```python
from build123d import *

# Parameters (mm, degrees)
AUFSATZ_LINEAR_AUSTRAGEN1_DEPTH = 5
VERRUNDUNG2_R                   = 2
SKIZZE7_R                       = 15
AUFSATZ_LINEAR_AUSTRAGEN3_DEPTH = 10
AUFSATZ_LINEAR_AUSTRAGEN5_DEPTH = 10
SCHNITT_LINEAR_AUSTRAGEN2_REACH = 17
SKIZZE9_R                       = 4
SCHNITT_LINEAR_AUSTRAGEN3_REACH = 7
SKIZZE10_R                      = 4


with BuildPart() as part:
    # Skizze1 → Aufsatz-Linear austragen1 (new body)
    with BuildSketch(Plane(origin=(0, 0, 0), x_dir=(0, 0, -1), z_dir=(1, 0, 0))):
        with BuildLine():
            Line((-20, 0), (-20, 45))
            Line((-20, 45), (-7, 55))
            Line((-7, 55), (7, 55))
            Line((7, 55), (20, 45))
            Line((20, 45), (20, 0))
            ThreePointArc((20, 0), (0, -20), (-20, 0))
        make_face()
    extrude(amount=-AUFSATZ_LINEAR_AUSTRAGEN1_DEPTH)

    # Verrundung2
    verrundung2_edges = [part.edges().sort_by_distance(p)[0] for p in [
        (-2.5, 45, 20),
        (-2.5, 55, 7),
        (-2.5, 55, -7),
        (-2.5, 45, -20),
    ]]
    fillet(verrundung2_edges, radius=VERRUNDUNG2_R)

    # Skizze7 → Aufsatz-Linear austragen3 (add)
    with BuildSketch(Plane.ZY.offset(5)):
        with Locations((0, 36)):
            Circle(SKIZZE7_R)
    extrude(amount=AUFSATZ_LINEAR_AUSTRAGEN3_DEPTH)

    # Skizze8 → Aufsatz-Linear austragen5 (add)
    with BuildSketch(Plane.ZY.offset(5)):
        with BuildLine():
            Line((15.909902577, 25.746951673), (10.253048327, 20.090097423))
            Line((10.253048327, 20.090097423), (8.126024025, 22.217121725))
            ThreePointArc((8.126024025, 22.217121725), (11.313708499, 24.686291501), (13.782878275, 27.873975975))
            Line((13.782878275, 27.873975975), (15.909902577, 25.746951673))
        make_face()
    aufsatz_linear_austragen5 = extrude(amount=AUFSATZ_LINEAR_AUSTRAGEN5_DEPTH)

    # Spiegeln2: Aufsatz-Linear austragen5 across plane
    add(aufsatz_linear_austragen5.mirror(Plane.XY))

    # Skizze9 → Schnitt-Linear austragen2 (cut, up to next)
    with BuildSketch(Plane.ZY.offset(15), mode=Mode.PRIVATE) as schnitt_linear_austragen2_sk1:
        with Locations((0, 36)):
            Circle(SKIZZE9_R)
    schnitt_linear_austragen2_tool1 = extrude(schnitt_linear_austragen2_sk1.sketch, amount=-SCHNITT_LINEAR_AUSTRAGEN2_REACH, mode=Mode.PRIVATE) & part.part
    add(schnitt_linear_austragen2_tool1.solids().sort_by_distance((-15, 36, 0))[0], mode=Mode.SUBTRACT)

    # Skizze10 → Schnitt-Linear austragen3 (cut, up to next)
    with BuildSketch(Plane.ZY.offset(5), mode=Mode.PRIVATE) as schnitt_linear_austragen3_sk1:
        Circle(SKIZZE10_R)
    schnitt_linear_austragen3_tool1 = extrude(schnitt_linear_austragen3_sk1.sketch, amount=-SCHNITT_LINEAR_AUSTRAGEN3_REACH, mode=Mode.PRIVATE) & part.part
    add(schnitt_linear_austragen3_tool1.solids().sort_by_distance((-5, 0, 0))[0], mode=Mode.SUBTRACT)


solid = part.part
```
Geometry check sheet. Reference: the model listing, model coordinates, mm. A direction names the side the tool comes from. Give positions to 0.01 mm unless a question says otherwise; leave off trailing zeros. Write each loop counter-clockwise with the first axis right and the second up, starting at its lowest first coordinate (ties: lowest second). Pieces come first, ordered by that corner, then holes.
1) Material ranges on L1, parallel to Y at x = -2.3, z = 0; L2, parallel to X at y = -4, z = -9.5; L3, parallel to Y at x = -5.75, z = -12, recorded low to high.
2) Section check B-B, the plane z = 0. Record the boundary of the cut face in (x, y).
3) Section check C-C, the plane y = 36. Record the boundary of the cut face in (x, z).
4) Access from +Z, -Z, +X, -X, +Y, -Y to the whole of each face (thin tool, end or side, straight path). Record for faces 1 (the flat face through (-9.93, 26.825, -14.832)), 2 (the flat face through (-9.93, 22.958, 13.121)), 3 (the flat face through (-9.93, 26.825, 14.832)), 4 (the cylindrical face through (-9.93, 50.872, -1.953)).
5) Section check A-A, the plane x = -13.25. Record the boundary of the cut face in (y, z).
6) Release check for a two-part mould opening along Y. For faces 5 (the cylindrical face through (-2.54, 44.89, 19.8)), 6 (the flat face through (0, 18, 0)), 7 (the cylindrical face through (-9.93, 24.646, 11.274)), 8 (the flat face through (-9.93, 22.958, -13.121)) record: pulls with the +Y half, pulls with the -Y half, needs draft (parallel to the pull), parting line crosses it, or undercut.
7) Section check D-D, the plane y = 27. Record the boundary of the cut face in (x, z).
8) Gauge pin test, flat ends, axial feed: pin 1 (1 mm diameter, centred on x = -3, z = 11, fed in from +Y); pin 2 (6 mm diameter, centred on x = -7.5, y = -5, fed in from +Z); pin 3 (8 mm diameter, centred on x = -5.5, z = -12, fed in from +Y); pin 4 (3 mm diameter, centred on y = 22.5, z = 12.5, fed in from +X). Record the tip position at first contact, or that the pin passes through.
Computed:
1. L1: y = -20 to -4, 4 to 32, 40 to 55
1. L2: x = -5 to 0
1. L3: y = 21.84 to 25.42, 27 to 45
2. outline: (-15, 21) - (-5, 21) - (-5, 4) - (0, 4) - (0, 32) - (-15, 32) - close; (-15, 40) - (0, 40) - (0, 55) - (-5, 55) - (-5, 51) - (-15, 51) - close; (-5, -20) - (0, -20) - (0, -4) - (-5, -4) - close
3. outline: (-15, -15) - (-5, -15) - (-5, -20) - (0, -20) - (0, -4) - (-15, -4) - close; (-15, 4) - (0, 4) - (0, 20) - (-5, 20) - (-5, 15) - (-15, 15) - close
4. face 1: -Z, -X
4. face 2: +Z, -X, -Y
4. face 3: +Z, -X
4. face 4: -X
5. outline: (20.09, -10.25) - (25.75, -15.91) - (27.87, -13.78) arc R16 cw to (22.22, -8.13) - close; (20.09, 10.25) - (22.22, 8.13) arc R16 cw to (27.87, 13.78) - (25.75, 15.91) - close; circle Ø30 at (36, 0); hole circle Ø8 at (36, 0)
6. face 5: pulls with the +Y half
6. face 6: needs draft
6. face 7: undercut
6. face 8: pulls with the -Y half
7. outline: (-15, -14.66) - (-5, -14.66) - (-5, -20) - (0, -20) - (0, 20) - (-5, 20) - (-5, 14.66) - (-15, 14.66) - (-15, 13.23) - (-5, 13.23) - (-5, 12) - (-15, 12) - (-15, -12) - (-5, -12) - (-5, -13.23) - (-15, -13.23) - close
8. pin 1: stops at y = 52.31
8. pin 2: stops at z = 19.72
8. pin 3: stops at y = 54.21
8. pin 4: stops at x = 0
